from build123d import *

# Parameters (mm, degrees)
SKETCH1_R           = 34.925
BOSS_EXTRUDE1_DEPTH = 1.27
SKETCH3_R           = 11.303
CUT_EXTRUDE1_DEPTH  = 6.35
CIRPATTERN1_COUNT   = 9
FILLET1_R           = 1.27
SKETCH5_R           = 1.5875
CUT_EXTRUDE2_DEPTH  = 6.35
SKETCH6_R           = 1.27
CUT_EXTRUDE3_DEPTH  = 49.864387552


with BuildPart() as part:
    # Sketch1 → Boss-Extrude1 (new, symmetric)
    with BuildSketch(Plane(origin=(0, 0, 0), x_dir=(0, 0, -1), z_dir=(1, 0, 0))):
        Circle(SKETCH1_R)
    extrude(amount=BOSS_EXTRUDE1_DEPTH, both=True)

    # Sketch3 → Cut-Extrude1 (cut, symmetric)
    with BuildSketch(Plane(origin=(0, 0, 0), x_dir=(0, 0, -1), z_dir=(1, 0, 0))):
        with Locations((0, -34.925)):
            Circle(SKETCH3_R)
    cut_extrude1 = extrude(amount=CUT_EXTRUDE1_DEPTH, both=True, mode=Mode.SUBTRACT)

    # CirPattern1: Cut-Extrude1 ×9 about axis
    cirpattern1_axis = Axis((0, 0, 0), (1, 0, 0))
    for i in range(1, CIRPATTERN1_COUNT):
        add(cut_extrude1.rotate(cirpattern1_axis, i * 360 / CIRPATTERN1_COUNT), mode=Mode.SUBTRACT)

    # Fillet1
    # the kernel refuses this fillet: 1.27 mm, written as the material it takes off along each edge
    with BuildSketch(Plane(origin=(-4.923134512, -16.731633019, -30.656289429), x_dir=(0, 0.38689872135285164, 0.9221222150103143), z_dir=(1, 0, 0)), Plane(origin=(-4.923134512, 27.285133925, -21.800850711), x_dir=(0, -0.8409288486623601, 0.541145702641532), z_dir=(1, 0, 0)), Plane(origin=(-4.923134512, 34.91494194, 0.838125473), x_dir=(0, -0.9920306242693342, -0.12599698612187168), z_dir=(1, 0, 0)), Plane(origin=(-4.923134512, 26.207660586, 23.084933434), x_dir=(0, -0.6789502455883892, -0.7341842847783286), z_dir=(1, 0, 0)), Plane(origin=(-4.923134512, 5.237523577, 34.53004448), x_dir=(0, -0.048181501305167504, -0.9988385970375695), z_dir=(1, 0, 0)), Plane(origin=(-4.923134512, -18.183308922, 29.818163955), x_dir=(0, 0.6051319029164822, -0.7961252288884437), z_dir=(1, 0, 0)), Plane(origin=(-4.923134512, -33.095969091, 11.154033124), x_dir=(0, 0.9752973644715361, -0.22089601819606364), z_dir=(1, 0, 0)), Plane(origin=(-4.923134512, -32.522657502, -12.729193769), x_dir=(0, 0.8891103499675269, 0.45769289439603716), z_dir=(1, 0, 0))) as fillet1_piece_1:
        with BuildLine():
            CenterArc((1.436473101, 1.267699411), FILLET1_R, 171.739357487, 94.811422393)
            ThreePointArc((0.179649711, 1.450168495), (0.082239687, 0.726023913), (0, 0))
            ThreePointArc((0, 0), (0.680032479, 0.020475246), (1.360064958, 0))
        make_face()
    extrude(amount=9.846269024, mode=Mode.SUBTRACT)
    with BuildSketch(Plane(origin=(-4.923134512, 5.237523577, -34.53004448), x_dir=(0, 0.9853377060596639, 0.1706153715732537), z_dir=(1, 0, 0)), Plane(origin=(-4.923134512, 34.91494194, -0.838125473), x_dir=(0, 0.0030787563353731583, 0.999995260618483), z_dir=(1, 0, 0)), Plane(origin=(-4.923134512, 27.285133925, 21.800850711), x_dir=(0, -0.6404260990883884, 0.7680197989677282), z_dir=(1, 0, 0)), Plane(origin=(-4.923134512, 6.888308505, 34.238966558), x_dir=(0, -0.984268465205427, 0.17667933779067993), z_dir=(1, 0, 0)), Plane(origin=(-4.923134512, -16.731633019, 30.656289429), x_dir=(0, -0.8675606775273359, -0.497331349110741), z_dir=(1, 0, 0)), Plane(origin=(-4.923134512, -32.522657502, 12.729193769), x_dir=(0, -0.34491160697127204, -0.9386351705409801), z_dir=(1, 0, 0)), Plane(origin=(-4.923134512, -18.183308922, -29.818163955), x_dir=(0, 0.8644819211919598, -0.5026639115077373), z_dir=(1, 0, 0))) as fillet1_piece_2:
        with BuildLine():
            CenterArc((1.434685554, 1.269722067), FILLET1_R, 176.387286037, 94.811422393)
            ThreePointArc((0.167209335, 1.349747283), (0.103924585, 0.67235637), (0, 0))
            ThreePointArc((0, 0), (0.730626902, -0.007643151), (1.461253805, 0))
        make_face()
    extrude(amount=9.846269024, mode=Mode.SUBTRACT)
    with BuildSketch(Plane(origin=(-4.923134512, 6.888308505, -34.238966558), x_dir=(0, -0.984268465205427, -0.1766793377906796), z_dir=(1, 0, 0))) as fillet1_piece_3:
        with BuildLine():
            CenterArc((1.434685554, -1.269722067), FILLET1_R, 88.80129157, 94.811422393)
            ThreePointArc((0.167209335, -1.349747283), (0.103924585, -0.67235637), (0, 0))
            ThreePointArc((0, 0), (0.730626902, 0.007643151), (1.461253805, 0))
        make_face()
    extrude(amount=9.846269024, mode=Mode.SUBTRACT)
    with BuildSketch(Plane(origin=(-4.923134512, 26.207660586, -23.084933434), x_dir=(0, -0.6789502455883865, 0.7341842847783312), z_dir=(1, 0, 0)), Plane(origin=(-4.923134512, -33.095969091, -11.154033124), x_dir=(0, 0.9752973644715363, 0.22089601819606305), z_dir=(1, 0, 0))) as fillet1_piece_4:
        with BuildLine():
            CenterArc((1.436473101, -1.267699411), FILLET1_R, 93.44922012, 94.811422393)
            ThreePointArc((0.179649711, -1.450168495), (0.082239687, -0.726023913), (0, 0))
            ThreePointArc((0, 0), (0.680032479, -0.020475246), (1.360064958, 0))
        make_face()
    extrude(amount=9.846269024, mode=Mode.SUBTRACT)

    # Sketch5 → Cut-Extrude2 (cut, symmetric)
    with BuildSketch(Plane(origin=(0, 0, 0), x_dir=(0, 0, -1), z_dir=(1, 0, 0))):
        Circle(SKETCH5_R)
    extrude(amount=CUT_EXTRUDE2_DEPTH, both=True, mode=Mode.SUBTRACT)

    # Sketch6 → Cut-Extrude3 (cut, through all)
    with BuildSketch(Plane(origin=(1.27, 0, 0), x_dir=(0, 0, -1), z_dir=(1, 0, 0))):
        with Locations((-5.5, 0)):
            Circle(SKETCH6_R)
        with Locations((5.5, 0)):
            Circle(SKETCH6_R)
    extrude(amount=-CUT_EXTRUDE3_DEPTH, mode=Mode.SUBTRACT)


solid = part.part
The model under review builds one solid part; all positions refer to its coordinate system, in mm. Give positions to 0.01 mm unless a question says otherwise; leave off trailing zeros. Order: outer loops, then holes, each group sorted by start corner. A loop starts at its lowest first (then second) coordinate and runs counter-clockwise, first axis right, second up. Notation, with made-up numbers: M 12,51.5 L 34,51.5 A23 cw 34,86.5 Z; hole C 58,-29.5 d4. An arc over 180 degrees is marked long. One line per question, with ' | ' between items. Start each with the question number.
1) Consider section B-B, the plane z = -5.5. Give the boundary of the cut face in (x, y), then the cut area to 3 significant figures.
2) Mouldability with a two-part tool opening along Y and no side actions: class faces 1 (the face through (0.018, -23.624, -0.204)), 2 (the face through (-1.27, 2, 0)), 3 (the face through (0.02, -1.55, 0.34)) as pulls with the +Y half, pulls with the -Y half, needs draft (parallel to the pull), parting line crosses it, or undercut.
3) Consider section C-C, the plane y = 0. Give the boundary of the cut face in (x, z).
4) Clearance check with a flat-ended pin moving along its axis: P1, Ø1.5, axis at x = -0.5, z = 5, coming from the -Y side. State where the tip first meets the part, or that it passes through.
5) Wall thickness on L1, parallel to Z at x = -0.3, y = 25; L2, parallel to Y at x = 1.05, z = -28.5; L3, parallel to Y at x = -0.55, z = 5.5: over which ranges is each line inside the solid? List them lowest first. Write a range as from..to.
6) Consider section A-A, the plane y = 23. Give the boundary of the cut face in (x, z).
7) Consider section D-D, the plane x = -0.5. State how many separate pieces and enclosed holes the cut face has, then the cut area to 3 significant figures.
Found:
1) outline: M -1.27,-25.05 L 1.27,-25.05 L 1.27,-1.27 L -1.27,-1.27 Z; M -1.27,1.27 L 1.27,1.27 L 1.27,23.53 L -1.27,23.53 Z | area: 117 mm²
2) face 1: pulls with the -Y half | face 2: needs draft | face 3: undercut
3) outline: M -1.27,-24.86 L 1.27,-24.86 L 1.27,-6.77 L -1.27,-6.77 Z; M -1.27,-4.23 L 1.27,-4.23 L 1.27,-1.59 L -1.27,-1.59 Z; M -1.27,1.59 L 1.27,1.59 L 1.27,4.23 L -1.27,4.23 Z; M -1.27,6.77 L 1.27,6.77 L 1.27,24.86 L -1.27,24.86 Z
4) P1: stops at y = -25.19
5) L1: z = -21.82..-20.11, -3.78..3.78, 20.11..21.82 | L2: y = -17.21..-15.71, 3.58..6.3 | L3: y = -25.05..-1.27, 1.27..23.53
6) outline: M -1.27,-20.39 L 1.27,-20.39 L 1.27,-17.54 L -1.27,-17.54 Z; M -1.27,-6.35 L 1.27,-6.35 L 1.27,6.35 L -1.27,6.35 Z; M -1.27,17.54 L 1.27,17.54 L 1.27,20.39 L -1.27,20.39 Z
7) separate pieces: 1 | enclosed holes: 3 | area: 2,120 mm²
